The model under review builds one solid part; all positions refer to its coordinate system, in mm. Face numbers are marked on the shaded views. A direction names the side the tool comes from. Coordinates: 2 decimals unless noted, no trailing zeros. Order: outer loops, then holes, each group sorted by start corner. A loop starts at its lowest first (then second) coordinate and runs counter-clockwise, first axis right, second up. Notation, with made-up numbers: (71.25, -27) -> (85.25, -27) arc R25 ccw to (85.25, 5) -> close; hole circle Ø9 at (48.5, 68). An arc over 180 degrees is marked (long way). Put each result on its own line as item: value.
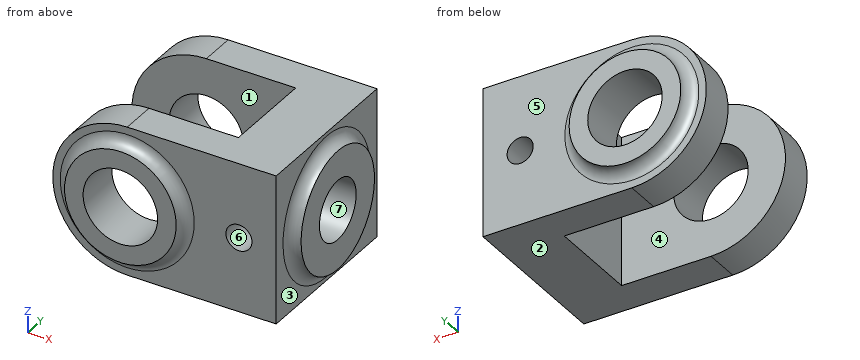
Autodesk Inventor part; units mm, degrees
ref_plane "YZ Plane" through (0, 0, 0) normal (1, 0, 0) x (0, 1, 0)
ref_plane "XZ Plane" through (0, 0, 0) normal (0, 1, 0) x (-1, 0, 0)
ref_plane "XY Plane" through (0, 0, 0) normal (0, 0, 1) x (1, 0, 0)
sketch "Szkic1" plane through (0, 0, 0) normal (0, 1, 0) x (-1, 0, 0)
  line L0 (0, 10.6544) -> (0, -29.3456)
  line L1 (0, -29.3456) -> (40, -29.3456)
  line L2 (0, 10.6544) -> (40, 10.6544)
  arc A0 (40, -29.3456) -> (40, 10.6544) centre (40, -9.3456) ccw
  point P0 (0, 0)
  dimension "d0" = 40
  dimension "d1" = 40
extrude "Wyciągnięcie proste1" add sketch "Szkic1" along normal blind 9.5
sketch "Szkic2" plane through (0, 9.5, 0) normal (0, 1, 0) x (1, 0, 0)
  line L0 (-40, -10.6544) -> (0, -10.6544)
  line L1 (0.0007, -10.6544) -> (-40, -10.6544)
  arc A0 (-40, 29.3456) -> (-40, -10.6544) centre (-40, 9.3456) ccw
  circle A1 centre (-40, 9.3456) radius 15
  circle A2 centre (-40, 9.3456) radius 10
  point P0 (0, 0)
  dimension "d4" = 30
  dimension "d5" = 20
extrude "Wyciągnięcie proste2" add sketch "Szkic2" along normal blind 3
fillet "Zaokrąglenie1" radius 3 1 edges at (-55, 9.5, -9.3456)
sketch "Szkic3" plane through (0, 0, 0) normal (0, -1, 0) x (1, 0, 0)
  line L0 (0, 10.6544) -> (0, -29.3456)
  line L1 (0, -29.3456) -> (-16, -29.3456)
  line L2 (0, -29.3456) -> (-40, -29.3456)
  line L3 (-16, -29.3456) -> (-16, 10.6544)
  line L4 (-40, 10.6544) -> (0, 10.6544)
  line L5 (-16, 10.6544) -> (0, 10.6544)
  line L6 (0, 10.6544) -> (0, -29.3456)
  point P0 (0, 0)
  dimension "d9" = 16
  dimension "d10" = 40
extrude "Wyciągnięcie proste3" add sketch "Szkic3" along normal blind 12.5
sketch "Szkic4" plane through (-40, 9.5, -9.3456) normal (0, 1, 0) x (1, 0, 0)
  point P0 (40, -9.3456)
mirror "Odbij1" about plane through (-8, -12.5, -9.3456) normal (0, -1, 0)
sketch "Szkic7" plane through (0, 9.5, 10.6544) normal (1, 0, 0) x (0, 0, -1)
  point P0 (10.6544, -9.5)
sketch "Szkic8" plane through (0, 9.5, 10.6544) normal (1, 0, 0) x (0, 0, -1)
  point P0 (10.6544, -9.5)
sketch "Szkic9" plane through (0, 9.5, 10.6544) normal (1, 0, 0) x (0, 0, -1)
  line L0 (40, 0) -> (0, 0)
  line L1 (0, 0) -> (0, -22)
  line L2 (0, -44) -> (0, 0)
  line L3 (0, -22) -> (20, -22)
  circle A0 centre (20, -22) radius 16
  circle A1 centre (20, -22) radius 8
  point P0 (10.6544, -9.5)
  dimension "d15" = 22
  dimension "d16" = 32
  dimension "d17" = 16
extrude "Wyciągnięcie proste4" cut sketch "Szkic9" against normal blind 20 contours A1
sketch "Szkic10" plane through (0, 9.5, 10.6544) normal (1, 0, 0) x (0, 0, -1)
  line L0 (0, -9.5) -> (0, 0)
  line L1 (0, 0) -> (0, -22)
  line L2 (0, -22) -> (20, -22)
  circle A0 centre (20, -22) radius 16
  point P0 (10.6544, -9.5)
  dimension "d20" = 22
  dimension "d21" = 20
  dimension "d22" = 32
extrude "Wyciągnięcie proste5" add sketch "Szkic10" along normal blind 3
fillet "Zaokrąglenie2" radius 3 1 edges at (0, -12.5, 6.6544)
sketch "Szkic11" plane through (3, -12.5, -9.3456) normal (1, 0, 0) x (0, 0, -1)
  circle A0 centre (0, 0) radius 8
  point P0 (-9.3456, 12.5)
  dimension "d26" = 16
extrude "Wyciągnięcie proste6" cut sketch "Szkic11" against normal blind 20
sketch "Szkic12" plane through (0, 0, 0) normal (0, -1, 0) x (1, 0, 0)
  point P0 (0, 0)
sketch "Szkic13" plane through (-40, -34.5, -9.3456) normal (0, -1, 0) x (1, 0, 0)
  point P0 (40, 9.3456)
sketch "Szkic14" plane through (-40, 12.5, -9.3456) normal (0, 1, 0) x (1, 0, 0)
  point P0 (40, -9.3456)
sketch "Szkic15" plane through (-40, 9.5, -9.3456) normal (0, 1, 0) x (1, 0, 0)
  circle A0 centre (0, 0) radius 10
  point P0 (40, -9.3456)
  dimension "d29" = 20
extrude "Wyciągnięcie proste7" cut sketch "Szkic15" against normal blind 9.5
sketch "Szkic16" plane through (-40, -34.5, -9.3456) normal (0, -1, 0) x (1, 0, 0)
  circle A0 centre (0, 0) radius 10
  point P0 (40, 9.3456)
  dimension "d32" = 20
extrude "Wyciągnięcie proste8" cut sketch "Szkic16" against normal blind 9.5
sketch "Szkic17" plane through (0, 9.5, 0) normal (0, 1, 0) x (1, 0, 0)
  line L0 (0, -10.6544) -> (0, 29.3456)
  line L1 (0, 9.3456) -> (-10, 9.3456)
  point P0 (0, 0)
hole "Otwór1" at (-10, 9.5, -9.3456) direction (0, -1, 0) diameter 7 depth 75.75 tip angle 118
properties part number "nakrętka" material "Stal nierdzewna, austenityczna"
Item 1: Consider section C-C on x = -4.5. Write out the cut boundary in (y, z), and give its area (3 significant figures).
Answers below:
outline: (-34.5, -29.35) -> (9.5, -29.35) -> (9.5, 10.65) -> (-34.5, 10.65) -> close; hole circle Ø16 at (-12.5, -9.35)
area: 1,560 mm^2
Item 2: Consider section D-D on z = -14. Count the separate pieces of the cut face and the enclosed holes in it, and give its area (3 significant figures).
Answers below:
separate pieces: 4
enclosed holes: 0
area: 1,110 mm^2
Item 3: For the marked faces 1, 2 and 3, list the 3-axis set-ups (+Z, -Z, +X, -X, +Y, -Y) from which the entire face can be reached by the end or side of a thin tool; tool diameter is ignored.
Answers below:
face 1: +Z, -Z, -X
face 2: -Z, +X, -X, +Y, -Y
face 3: +X
Item 4: For line 1 (Z direction, x = -8, y = -12.5); line 2 (Y direction, x = -37, z = -21); line 3 (Z direction, x = -10, y = -22.75), list the stretches that pass through material, from the lowest coordinate up. Write a range as from..to.
Answers below:
line 1: -29.35..-17.35, -1.35..10.65
line 2: -37.5..-25, 0..12.5
line 3: -29.35..-12.85, -5.85..10.65
Item 5: Consider section B-B on x = -17. Write out the cut boundary in (y, z).
Answers below:
outline: (-34.5, -29.35) -> (-25, -29.35) -> (-25, 10.65) -> (-34.5, 10.65) -> close; (0, -29.35) -> (9.5, -29.35) -> (9.5, 10.65) -> (0, 10.65) -> close
Item 6: For pin 1 Ø4 at (y, z) = (-15, -14) entering from +X; pin 2 Ø20 at (x, z) = (-34.5, -6.5) entering from +Y; pin 3 Ø5 at (x, z) = (-19.5, -17) entering from -Y; pin 4 Ø20 at (y, z) = (-16.5, -12.5) entering from -X, all flat-tipped, find the tip position at first contact; note any pin that passes through.
Answers below:
pin 1: through
pin 2: y = 12.5
pin 3: y = -34.5
pin 4: x = -60
Item 7: Mouldability with a two-part tool opening along Y and no side actions: class the marked faces 4, 5, 6 and 7 as +Y half, -Y half, draft (parallel to the pull), parting line (faces both ways), or undercut.
Answers below:
face 4: undercut
face 5: +Y half
face 6: draft
face 7: undercut
